```python
from build123d import *

# Parameters (mm, degrees)
EXTRUDE_1_DEPTH     = 35
SKETCH_5_R          = 17.5
CUT_EXTRUDE_3_DEPTH = 27.5
SKETCH_6_R          = 18.6
CUT_EXTRUDE_4_DEPTH = 3
CUT_EXTRUDE_5_DEPTH = 6.48
CUT_EXTRUDE_6_DEPTH = 55.049209838
EXTRUDE_START       = 5.52
EXTRUDE_2_DEPTH     = 5.52
SKETCH_12_R         = 1.3
CUT_EXTRUDE_7_DEPTH = 55.049209838
SKETCH_13_R         = 17.5
SKETCH_13_R_2       = 1.3
EXTRUDE_3_DEPTH     = 2


with BuildPart() as part:
    # 草图1 → 凸台-拉伸1 (new body)
    with BuildSketch(Plane(origin=(0, 0, 0), x_dir=(1, 0, 0), z_dir=(0, 1, 0))):
        with BuildLine():
            Line((13.565756947, 31.180270004), (15.409458345, 30.41658388))
            ThreePointArc((15.409458345, 30.41658388), (15.890161366, 29.821935938), (15.652026017, 29.095318346))
            ThreePointArc((15.652026017, 29.095318346), (12.665907923, 22.315459341), (15.450283169, 15.450283169))
            ThreePointArc((15.450283169, 15.450283169), (21.486135899, 12.444530691), (28.114304746, 13.682853695))
            ThreePointArc((28.114304746, 13.682853695), (30.152483097, 13.859644928), (31.640219088, 12.45534163))
            Line((31.640219088, 12.45534163), (32.403905212, 10.611640232))
            ThreePointArc((32.403905212, 10.611640232), (32.323333986, 9.851252274), (31.641150639, 9.505843167))
            ThreePointArc((31.641150639, 9.505843167), (24.735562008, 6.823263243), (21.85, 0))
            ThreePointArc((21.85, 0), (23.992604436, -6.393380355), (29.555054168, -10.2045769))
            ThreePointArc((29.555054168, -10.2045769), (31.121274181, -11.520776354), (31.180270004, -13.565756947))
            Line((31.180270004, -13.565756947), (30.41658388, -15.409458345))
            ThreePointArc((30.41658388, -15.409458345), (29.821935938, -15.890161366), (29.095318346, -15.652026017))
            ThreePointArc((29.095318346, -15.652026017), (22.315459341, -12.665907923), (15.450283169, -15.450283169))
            ThreePointArc((15.450283169, -15.450283169), (12.444530691, -21.486135899), (13.682853695, -28.114304746))
            ThreePointArc((13.682853695, -28.114304746), (13.859644928, -30.152483097), (12.45534163, -31.640219088))
            Line((12.45534163, -31.640219088), (10.611640232, -32.403905212))
            ThreePointArc((10.611640232, -32.403905212), (9.851252274, -32.323333986), (9.505843167, -31.641150639))
            ThreePointArc((9.505843167, -31.641150639), (6.823263243, -24.735562008), (0, -21.85))
            ThreePointArc((0, -21.85), (-6.393380355, -23.992604436), (-10.2045769, -29.555054168))
            ThreePointArc((-10.2045769, -29.555054168), (-11.520776354, -31.121274181), (-13.565756947, -31.180270004))
            Line((-13.565756947, -31.180270004), (-15.409458345, -30.41658388))
            ThreePointArc((-15.409458345, -30.41658388), (-15.890161366, -29.821935938), (-15.652026017, -29.095318346))
            ThreePointArc((-15.652026017, -29.095318346), (-12.665907923, -22.315459341), (-15.450283169, -15.450283169))
            ThreePointArc((-15.450283169, -15.450283169), (-21.486135899, -12.444530691), (-28.114304746, -13.682853695))
            ThreePointArc((-28.114304746, -13.682853695), (-30.152483097, -13.859644928), (-31.640219088, -12.45534163))
            Line((-31.640219088, -12.45534163), (-32.403905212, -10.611640232))
            ThreePointArc((-32.403905212, -10.611640232), (-32.323333986, -9.851252274), (-31.641150639, -9.505843167))
            ThreePointArc((-31.641150639, -9.505843167), (-24.735562008, -6.823263243), (-21.85, 0))
            ThreePointArc((-21.85, 0), (-23.992604436, 6.393380355), (-29.555054168, 10.2045769))
            ThreePointArc((-29.555054168, 10.2045769), (-31.121274181, 11.520776354), (-31.180270004, 13.565756947))
            Line((-31.180270004, 13.565756947), (-30.41658388, 15.409458345))
            ThreePointArc((-30.41658388, 15.409458345), (-29.821935938, 15.890161366), (-29.095318346, 15.652026017))
            ThreePointArc((-29.095318346, 15.652026017), (-22.315459341, 12.665907923), (-15.450283169, 15.450283169))
            ThreePointArc((-15.450283169, 15.450283169), (-12.444530691, 21.486135899), (-13.682853695, 28.114304746))
            ThreePointArc((-13.682853695, 28.114304746), (-13.859644928, 30.152483097), (-12.45534163, 31.640219088))
            Line((-12.45534163, 31.640219088), (-10.611640232, 32.403905212))
            ThreePointArc((-10.611640232, 32.403905212), (-9.851252274, 32.323333986), (-9.505843167, 31.641150639))
            ThreePointArc((-9.505843167, 31.641150639), (-6.823263243, 24.735562008), (0, 21.85))
            ThreePointArc((0, 21.85), (6.393380355, 23.992604436), (10.2045769, 29.555054168))
            ThreePointArc((10.2045769, 29.555054168), (11.520776354, 31.121274181), (13.565756947, 31.180270004))
        make_face()
    extrude(amount=EXTRUDE_1_DEPTH)

    # 草图5 → 切除-拉伸3 (cut)
    with BuildSketch(Plane(origin=(0, 35, 0), x_dir=(1, 0, 0), z_dir=(0, 1, 0))):
        with Locations(Location((0, 0, 0), (0, 0, 270))):
            Circle(SKETCH_5_R)
    extrude(amount=-CUT_EXTRUDE_3_DEPTH, mode=Mode.SUBTRACT)

    # 草图6 → 切除-拉伸4 (cut)
    with BuildSketch(Plane(origin=(0, 35, 0), x_dir=(1, 0, 0), z_dir=(0, 1, 0))):
        with Locations(Location((0, 0, 0), (0, 0, 270))):
            Circle(SKETCH_6_R)
    extrude(amount=-CUT_EXTRUDE_4_DEPTH, mode=Mode.SUBTRACT)

    # 草图7 → 切除-拉伸5 (cut)
    with BuildSketch(Plane.XZ):
        with BuildLine():
            ThreePointArc((9.10421468, 28.61165958), (11.228658553, 26.845140252), (13.682853695, 28.114304746))
            ThreePointArc((13.682853695, 28.114304746), (12.444530691, 21.486135899), (15.450283169, 15.450283169))
            ThreePointArc((15.450283169, 15.450283169), (20.785800914, 12.766861919), (26.669150448, 13.793846573))
            ThreePointArc((26.669150448, 13.793846573), (26.92224132, 11.042520107), (29.555054168, 10.2045769))
            ThreePointArc((29.555054168, 10.2045769), (23.992604436, 6.393380355), (21.85, 0))
            ThreePointArc((21.85, 0), (23.725315416, -5.670246141), (28.61165958, -9.10421468))
            ThreePointArc((28.61165958, -9.10421468), (26.845140252, -11.228658553), (28.114304746, -13.682853695))
            ThreePointArc((28.114304746, -13.682853695), (21.486135899, -12.444530691), (15.450283169, -15.450283169))
            ThreePointArc((15.450283169, -15.450283169), (12.766861919, -20.785800914), (13.793846573, -26.669150448))
            ThreePointArc((13.793846573, -26.669150448), (11.042520107, -26.92224132), (10.2045769, -29.555054168))
            ThreePointArc((10.2045769, -29.555054168), (6.393380355, -23.992604436), (0, -21.85))
            ThreePointArc((0, -21.85), (-5.670246141, -23.725315416), (-9.10421468, -28.61165958))
            ThreePointArc((-9.10421468, -28.61165958), (-11.228658553, -26.845140252), (-13.682853695, -28.114304746))
            ThreePointArc((-13.682853695, -28.114304746), (-12.444530691, -21.486135899), (-15.450283169, -15.450283169))
            ThreePointArc((-15.450283169, -15.450283169), (-20.785800914, -12.766861919), (-26.669150448, -13.793846573))
            ThreePointArc((-26.669150448, -13.793846573), (-26.92224132, -11.042520107), (-29.555054168, -10.2045769))
            ThreePointArc((-29.555054168, -10.2045769), (-23.992604436, -6.393380355), (-21.85, 0))
            ThreePointArc((-21.85, 0), (-23.725315416, 5.670246141), (-28.61165958, 9.10421468))
            ThreePointArc((-28.61165958, 9.10421468), (-26.845140252, 11.228658553), (-28.114304746, 13.682853695))
            ThreePointArc((-28.114304746, 13.682853695), (-21.486135899, 12.444530691), (-15.450283169, 15.450283169))
            ThreePointArc((-15.450283169, 15.450283169), (-12.766861919, 20.785800914), (-13.793846573, 26.669150448))
            ThreePointArc((-13.793846573, 26.669150448), (-11.042520107, 26.92224132), (-10.2045769, 29.555054168))
            ThreePointArc((-10.2045769, 29.555054168), (-6.393380355, 23.992604436), (0, 21.85))
            ThreePointArc((0, 21.85), (5.670246141, 23.725315416), (9.10421468, 28.61165958))
        make_face()
    extrude(amount=-CUT_EXTRUDE_5_DEPTH, mode=Mode.SUBTRACT)

    # 草图8 → 切除-拉伸6 (cut, through all)
    with BuildSketch(Plane.XZ.offset(-6.48)):
        with BuildLine():
            Line((1.833030278, 2.5), (-1.833030278, 2.5))
            ThreePointArc((-1.833030278, 2.5), (0, -3.1), (1.833030278, 2.5))
        make_face()
    extrude(amount=-CUT_EXTRUDE_6_DEPTH, mode=Mode.SUBTRACT)

    # 草图11 → 凸台-拉伸2 (add)
    with BuildSketch(Plane.XZ.offset(EXTRUDE_START)):
        with BuildLine():
            Line((31.640219088, -12.45534163), (32.403905212, -10.611640232))
            ThreePointArc((32.403905212, -10.611640232), (32.323333986, -9.851252274), (31.641150639, -9.505843167))
            ThreePointArc((31.641150639, -9.505843167), (30.110166925, -9.427513844), (28.61165958, -9.10421468))
            ThreePointArc((28.61165958, -9.10421468), (27.475741438, -13.174877522), (31.640219088, -12.45534163))
        make_face()
        with BuildLine():
            Line((31.180270004, 13.565756947), (30.41658388, 15.409458345))
            ThreePointArc((30.41658388, 15.409458345), (29.821935938, 15.890161366), (29.095318346, 15.652026017))
            ThreePointArc((29.095318346, 15.652026017), (27.957362185, 14.624844247), (26.669150448, 13.793846573))
            ThreePointArc((26.669150448, 13.793846573), (28.744328326, 10.112237852), (31.180270004, 13.565756947))
        make_face()
        with BuildLine():
            Line((12.45534163, 31.640219088), (10.611640232, 32.403905212))
            ThreePointArc((10.611640232, 32.403905212), (9.851252274, 32.323333986), (9.505843167, 31.641150639))
            ThreePointArc((9.505843167, 31.641150639), (9.427513844, 30.110166925), (9.10421468, 28.61165958))
            ThreePointArc((9.10421468, 28.61165958), (13.174877522, 27.475741438), (12.45534163, 31.640219088))
        make_face()
        with BuildLine():
            Line((-13.565756947, 31.180270004), (-15.409458345, 30.41658388))
            ThreePointArc((-15.409458345, 30.41658388), (-15.890161366, 29.821935938), (-15.652026017, 29.095318346))
            ThreePointArc((-15.652026017, 29.095318346), (-14.624844247, 27.957362185), (-13.793846573, 26.669150448))
            ThreePointArc((-13.793846573, 26.669150448), (-10.112237852, 28.744328326), (-13.565756947, 31.180270004))
        make_face()
        with BuildLine():
            Line((-31.640219088, 12.45534163), (-32.403905212, 10.611640232))
            ThreePointArc((-32.403905212, 10.611640232), (-32.323333986, 9.851252274), (-31.641150639, 9.505843167))
            ThreePointArc((-31.641150639, 9.505843167), (-30.110166925, 9.427513844), (-28.61165958, 9.10421468))
            ThreePointArc((-28.61165958, 9.10421468), (-27.475741438, 13.174877522), (-31.640219088, 12.45534163))
        make_face()
        with BuildLine():
            Line((-31.180270004, -13.565756947), (-30.41658388, -15.409458345))
            ThreePointArc((-30.41658388, -15.409458345), (-29.821935938, -15.890161366), (-29.095318346, -15.652026017))
            ThreePointArc((-29.095318346, -15.652026017), (-27.957362185, -14.624844247), (-26.669150448, -13.793846573))
            ThreePointArc((-26.669150448, -13.793846573), (-28.744328326, -10.112237852), (-31.180270004, -13.565756947))
        make_face()
        with BuildLine():
            Line((-12.45534163, -31.640219088), (-10.611640232, -32.403905212))
            ThreePointArc((-10.611640232, -32.403905212), (-9.851252274, -32.323333986), (-9.505843167, -31.641150639))
            ThreePointArc((-9.505843167, -31.641150639), (-9.427513844, -30.110166925), (-9.10421468, -28.61165958))
            ThreePointArc((-9.10421468, -28.61165958), (-13.174877522, -27.475741438), (-12.45534163, -31.640219088))
        make_face()
        with BuildLine():
            Line((13.565756947, -31.180270004), (15.409458345, -30.41658388))
            ThreePointArc((15.409458345, -30.41658388), (15.890161366, -29.821935938), (15.652026017, -29.095318346))
            ThreePointArc((15.652026017, -29.095318346), (14.624844247, -27.957362185), (13.793846573, -26.669150448))
            ThreePointArc((13.793846573, -26.669150448), (10.112237852, -28.744328326), (13.565756947, -31.180270004))
        make_face()
    extrude(amount=-EXTRUDE_2_DEPTH)

    # 草图12 → 切除-拉伸7 (cut, through all)
    with BuildSketch(Plane.XZ.offset(-6.48)):
        with Locations(Location((10, 0, 0), (0, 0, 270))):
            Circle(SKETCH_12_R)
        with Locations(Location((0, -10, 0), (0, 0, 270))):
            Circle(SKETCH_12_R)
        with Locations(Location((-10, 0, 0), (0, 0, 270))):
            Circle(SKETCH_12_R)
    extrude(amount=-CUT_EXTRUDE_7_DEPTH, mode=Mode.SUBTRACT)

    # 草图13 → 凸台-拉伸3 (add)
    with BuildSketch(Plane(origin=(0, 7.5, 0), x_dir=(1, 0, 0), z_dir=(0, 1, 0))):
        with Locations(Location((0, 0, 0), (0, 0, 270))):
            Circle(SKETCH_13_R)
        with Locations(Location((-10, 0, 0), (0, 0, 90))):
            Circle(SKETCH_13_R_2, mode=Mode.SUBTRACT)
        with Locations(Location((0, 10, 0), (0, 0, 90))):
            Circle(SKETCH_13_R_2, mode=Mode.SUBTRACT)
        with Locations(Location((10, 0, 0), (0, 0, 90))):
            Circle(SKETCH_13_R_2, mode=Mode.SUBTRACT)
        with BuildLine():
            Line((-1.833030278, -2.5), (1.833030278, -2.5))
            ThreePointArc((1.833030278, -2.5), (0, 3.1), (-1.833030278, -2.5))
        make_face(mode=Mode.SUBTRACT)
    extrude(amount=EXTRUDE_3_DEPTH)


solid = part.part
```
The listing builds one solid part. Answer for the finished solid, in the listing's coordinates (mm). A direction names the side the tool comes from. Give positions to 0.01 mm unless a question says otherwise; leave off trailing zeros. Loops run counter-clockwise (first coordinate to the right, second up) from the corner with the lowest first, then second, coordinate; pieces in that order, holes last. Notation, with made-up numbers: (84, 82.5) - (132, 82.5) arc R14 ccw to (132, 101.5) - close; hole circle Ø4 at (-3, 51.5). An arc over 180 degrees is marked (long way). Return JSON: item names as keys, results as strings. Group by question number.
1. Straight lines are drawn through the part: line 1 (Z direction, x = 0, y = 7.05); line 2 (X direction, y = 7, z = 0); line 3 (Y direction, x = 3.5, z = -9.5). For each, find the intervals that lie inside material, in ascending order. Write a range as [from, to].
2. Determine the mould class of faces 1 (the flat face through (-32.017, 14.456, 11.546)), 2 (the flat face through (0, 8, 2.5)), 3 (the flat face through (-31, 14, -14)) for opening direction Z: pulls with the +Z half, pulls with the -Z half, needs draft (parallel to the pull), parting line crosses it, or undercut.
3. Find section B-B (x = -25). Write down the section's boundary in (y, z).
4. Given pin 1 Ø1.5 at (x, y) = (-9, 29.5) entering from -Z; pin 2 Ø10 at (x, y) = (-25, -1.5) entering from +Z; pin 3 Ø10.5 at (x, z) = (-3.5, -3.5) entering from +Y; pin 4 Ø2 at (x, z) = (10, 0) entering from +Y, each flat-ended and moving along its own axis, determine where each tip first touches the part or whether it passes through.
5. Find section C-C (z = 4.5). Write down the section's boundary in (x, y), then the cut area to 3 significant figures.
6. Which of the six approach directions +Z, -Z, +X, -X, +Y, -Y give full straight-line access (tool end or side, diameter ignored) to faces 4 (the cylindrical face through (23.94, 20.54, 6.32)), 5 (the cylindrical face through (6.32, 20.54, -23.94)), 6 (the cylindrical face through (5.59, 33.52, 17.74)), 7 (the flat face through (0, 6.48, -6))?
7. Find section A-A (z = -25.5). Write down the section's boundary in (x, y).
Verdict:
{
 "1": {"line 1": "z = [-21.85, -11.3], [-8.7, -3.1], [2.5, 21.85]", "line 2": "x = [-21.85, -11.3], [-8.7, -3.1], [3.1, 8.7], [11.3, 21.85]", "line 3": "y = [6.48, 9.5]"},
 "2": {"face 1": "pulls with the +Z half", "face 2": "undercut", "face 3": "pulls with the -Z half"},
 "3": {"outline": "(6.48, -13.09) - (35, -13.09) - (35, -7.54) - (6.48, -7.54) - close; (6.48, 7.07) - (35, 7.07) - (35, 12.54) - (6.48, 12.54) - close"},
 "4": {"pin 1": "stops at z = -32.24", "pin 2": "stops at z = 14", "pin 3": "stops at y = 9.5", "pin 4": "passes through"},
 "5": {"outline": "(-22.98, 6.48) - (22.85, 6.48) - (22.85, 35) - (18.05, 35) - (18.05, 32) - (16.91, 32) - (16.91, 9.5) - (-16.91, 9.5) - (-16.91, 32) - (-18.05, 32) - (-18.05, 35) - (-22.98, 35) - close", "area": "438 mm^2"},
 "6": {"face 4": "+X, +Y, -Y", "face 5": "-Z, +Y, -Y", "face 6": "+Y", "face 7": "-Y"},
 "7": {"outline": "(-12.65, 6.48) - (-7.49, 6.48) - (-7.49, 35) - (-12.65, 35) - close; (8.01, 6.48) - (13.27, 6.48) - (13.27, 35) - (8.01, 35) - close"}
}
